Input: part model. Units: mm. Frame: model coordinates. A direction names the side the tool comes from. Round coordinates to 2 decimals unless told otherwise and drop trailing zeros. Answer in a Markdown table with one row per item. Add a question column.
Q1. Mould query, pull axis Z, two halves, no side actions, for faces 1 (the face through (-243, 10, 111)), 2 (the face through (-256, 4, 111)), 3 (the face through (-265.387, 4.93, 134.757)). Classes: pulls with the +Z half, pulls with the -Z half, needs draft (parallel to the pull), parting line crosses it, or undercut.
Q2. Ray query, L1, parallel to X at y = 0.75, z = 117.5; L2, parallel to X at y = 6.5, z = -193.5; L3, parallel to X at y = 8, z = 216. Return the intervals inside material, ascending. Write a range as from..to.
Q3. Pin query (flat end, axial travel): pin 1 (3 mm diameter, centred on x = 325, y = 5.5, fed in from +Z); pin 2 (0.8 mm diameter, centred on y = 1, z = -0.5, fed in from -X); pin 3 (6 mm diameter, centred on x = -239.5, y = 4.5, fed in from -Z); pin 4 (14 mm diameter, centred on x = -81.5, z = -350, fed in from -Y). Return the tip coordinate at first contact, or that it passes through.
Q4. Reachability of faces 4 (the face through (-68, 4, -347)), 5 (the face through (-293, 0, -112)) from +Z, -Z, +X, -X, +Y, -Y: full face, straight path, thin tool, end or side. Return the list, or none.
```python
from build123d import *

# Parameters (mm, degrees)
SKETCH1_RX          = 355
SKETCH1_RY          = 265
BOSS_EXTRUDE1_DEPTH = 10
SKETCH2_RX          = 365
SKETCH2_RY          = 275
SKETCH2_RX_2        = 355
SKETCH2_RY_2        = 265
CUT_EXTRUDE1_DEPTH  = 4
CUT_EXTRUDE4_START  = -580
CUT_EXTRUDE4_DEPTH  = 10
CUT_EXTRUDE5_DEPTH  = 10


with BuildPart() as part:
    # Sketch1 → Boss-Extrude1 (new body)
    with BuildSketch(Plane(origin=(0, 0, 0), x_dir=(1, 0, 0), z_dir=(0, 1, 0))):
        with BuildLine():
            Line((-320, 50), (-320, 65))
            Line((-320, 65), (-312.170159719, 128.33520269))
            add(Edge.make_bspline(
                [(212.28214963, 202.588475219), (-232.721291269, 770.993291043), (-312.170159719, 128.33520269)],
                knots=[4.895798945, 4.895798945, 4.895798945, 7.074054013, 7.074054013, 7.074054013], degree=2, weights=[1, 0.463258742, 1]))
            Line((212.28214963, 202.588475219), (320, 65))
            Line((320, 65), (320, 50))
            Line((320, 50), (330, 50))
            Line((330, 50), (330, 20))
            Line((330, 20), (320, 20))
            Line((320, 20), (320, 0))
            Line((320, 0), (320, -20))
            Line((320, -20), (330, -20))
            Line((330, -20), (330, -50))
            Line((330, -50), (320, -50))
            Line((320, -50), (320, -65))
            Line((320, -65), (312.170159719, -128.33520269))
            add(Edge.make_bspline(
                [(-212.28214963, -202.588475219), (232.721291269, -770.993291043), (312.170159719, -128.33520269)],
                knots=[1.754206291, 1.754206291, 1.754206291, 3.932461359, 3.932461359, 3.932461359], degree=2, weights=[1, 0.463258742, 1]))
            Line((-212.28214963, -202.588475219), (-320, -65))
            Line((-320, -65), (-320, -50))
            Line((-320, -50), (-330, -50))
            Line((-330, -50), (-330, -20))
            Line((-330, -20), (-320, -20))
            Line((-320, -20), (-320, 0))
            Line((-320, 0), (-320, 20))
            Line((-320, 20), (-330, 20))
            Line((-330, 20), (-330, 50))
            Line((-330, 50), (-320, 50))
        make_face()
        with Locations(Location((0, 0), (0, 0, 120))):
            Ellipse(SKETCH1_RX, SKETCH1_RY, mode=Mode.SUBTRACT)
    extrude(amount=BOSS_EXTRUDE1_DEPTH)

    # Sketch2 → Cut-Extrude1 (cut)
    with BuildSketch(Plane.XZ):
        with Locations(Location((0, 0), (0, 0, 90))):
            Ellipse(SKETCH2_RX, SKETCH2_RY)
        with Locations(Location((0, 0), (0, 0, 90))):
            Ellipse(SKETCH2_RX_2, SKETCH2_RY_2, mode=Mode.SUBTRACT)
    extrude(amount=-CUT_EXTRUDE1_DEPTH, mode=Mode.SUBTRACT)

    # Sketch4 → Cut-Extrude4 (cut)
    with BuildSketch(Plane.ZY.offset(290).offset(CUT_EXTRUDE4_START)):
        with BuildLine():
            Line((-2.5, 0), (2.5, 0))
            ThreePointArc((2.5, 0), (0, 2.5), (-2.5, 0))
        make_face()
    extrude(amount=CUT_EXTRUDE4_DEPTH, mode=Mode.SUBTRACT)

    # Sketch5 → Cut-Extrude5 (cut)
    with BuildSketch(Plane(origin=(290, 0, 0), x_dir=(0, 0, -1), z_dir=(1, 0, 0))):
        with BuildLine():
            Line((-2.5, 0), (2.5, 0))
            ThreePointArc((2.5, 0), (0, 2.5), (-2.5, 0))
        make_face()
    extrude(amount=-CUT_EXTRUDE5_DEPTH, mode=Mode.SUBTRACT)


solid = part.part
```
Answer block:
| question | item | result |
|---|---|---|
| 1 | face 1 | needs draft |
| 1 | face 2 | undercut |
| 1 | face 3 | pulls with the +Z half |
| 2 | L1 | -278.9..-260.36, -250.06..-237.8, 288.46..313.51 |
| 2 | L2 | -297.36..-271.03, 187.6..219.4 |
| 2 | L3 | -201.39..-168.13, 261.26..288.61 |
| 3 | pin 1 | z = 50 |
| 3 | pin 2 | x = -320 |
| 3 | pin 3 | z = -293.33 |
| 3 | pin 4 | y = 0 |
| 4 | face 4 | -Y |
| 4 | face 5 | +Z, -Z, +X, -X, -Y |
